Autodesk Inventor part; units mm, degrees
ref_plane "YZ Plane" through (0, 0, 0) normal (1, 0, 0) x (0, 1, 0)
ref_plane "XZ Plane" through (0, 0, 0) normal (0, 1, 0) x (-1, 0, 0)
ref_plane "XY Plane" through (0, 0, 0) normal (0, 0, 1) x (1, 0, 0)
sketch "Skizze2" plane through (0, 0, 0) normal (1, 0, 0) x (0, 1, 0)
  line L0 (0, 0) -> (18.8, 0)
  line L1 (0, 3.1) -> (3, 3.1)
  line L2 (18.8, 31.354) -> (17.3, 31.9)
  line L3 (17.3, 31.9) -> (14.3, 31.9)
  line L4 (14.3, 31.9) -> (14.3, 30.15)
  line L5 (14.3, 30.15) -> (10.8, 30.15)
  line L6 (10.8, 30.15) -> (10.8, 31.9)
  line L7 (10.8, 31.9) -> (7.8, 31.9)
  line L8 (7.8, 31.9) -> (7.8, 35)
  line L9 (7.8, 35) -> (0, 35)
  line L10 (18.8, 31.354) -> (18.8, 27)
  line L11 (18.8, 27) -> (3, 27)
  line L12 (3, 27) -> (3, 3.1)
  line L13 (0, 35) -> (0, 3.1)
  dimension "d5" = 6.2
  dimension "d10" = 20
  dimension "d11" = 60.3
  dimension "d12" = 63.8
  dimension "d26" = 70
  dimension "d34" = 1.5
  dimension "d35" = 4.5
  dimension "d36" = 8
  dimension "d37" = 11
  dimension "d39" = 3
  dimension "d41" = 18.8
  dimension "d50" = 54
revolve "Umdrehung1" add sketch "Skizze2" angle 360 about axis through (0, 0, 0) along (0, 1, 0)
fillet "Rundung1" radius 0.4 2 edges at (0, 10.8, -30.15) (0, 14.3, -30.15)
chamfer "Fase1" distance 0.5 angle 45 1 edges at (0, 0, -3.1)
sketch "Skizze7" plane through (0, 3, 0) normal (0, 1, 0) x (1, 0, 0)
  arc A0 (-7.5, -18.4326) -> (7.5, -18.4326) centre (0, 0) ccw
  circle A1 centre (0, 0) radius 31.9
  line L0 (0, 49) -> (0, -49)
  line L1 (-7.5, -18.4326) -> (-7.5, -25.9374)
  circle A2 centre (0, 0) radius 27
  line L2 (7.5, -18.4326) -> (7.5, -25.9374)
  arc A3 (-7.5, -25.9374) -> (7.5, -25.9374) centre (0, 0) ccw
  line L3 (7.5, 18.4326) -> (7.5, 25.9374)
  arc A4 (7.5, 18.4326) -> (-7.5, 18.4326) centre (0, 0) ccw
  arc A5 (7.5, 25.9374) -> (-7.5, 25.9374) centre (0, 0) ccw
  line L4 (-7.5, 18.4326) -> (-7.5, 25.9374)
  dimension "d70" = 12
  dimension "d73" = 360
  dimension "d75" = 15
extrude "Extrusion2" add sketch "Skizze7" along normal blind 10 contours A0 L0 A2 L1 | A0 L2 A2 L0 | A4 L4 A2 L0 | L0 A2 L3 A4
sketch "Skizze8" plane through (0, 13, 0) normal (0, 1, 0) x (1, 0, 0)
  line L0 (0, 49) -> (0, -49)
  point P0 (0, 0)
  point P1 (0, -23.5)
  dimension "d78" = 23.5
hole "Bohrung3" at (0, 13, 23.5) direction (0, -1, 0) diameter 2.5 depth 8 tip angle 118
thread "Gewinde1"
pattern_circular "Runde Anordnung1" count 2 over 360 about axis through (0, 10.9, 0) along (0, 1, 0) of "Bohrung3"
sketch "Skizze9" plane through (0, 0, 0) normal (0, -1, 0) x (1, 0, 0)
  line L0 (-49, 0) -> (49, 0)
  point P0 (0, 0)
  point P1 (-22, -8)
  point P2 (-22, 8)
  dimension "d91" = 16
  dimension "d92" = 22
hole "Bohrung4" at (-22, 0, -8) at (-22, 0, 8) direction (0, 1, 0) diameter 3.3 end through all
thread "Gewinde2"
thread "Gewinde3"
sketch "Skizze10" plane through (0, 13, 0) normal (0, 1, 0) x (1, 0, 0)
  point P0 (0, 0)
  point P1 (4, -23.5)
  dimension "d104" = 23.5
  dimension "d105" = 4
hole "Bohrung5" at (4, 13, 23.5) direction (0, -1, 0) diameter 0.8 end through all
hole "Bohrung6" at (4, 0, 23.5) direction (0, 1, 0) diameter 1.6 depth 5 tip angle 118
thread "Gewinde4"
sketch "Skizze11" plane through (0, 3, 0) normal (0, 1, 0) x (1, 0, 0)
  line L0 (-49, 0) -> (49, 0)
  point P0 (0, 0)
  point P1 (18.4, 0)
  dimension "d124" = 18.4
hole "Bohrung7" at (18.4, 3, 0) direction (0, -1, 0) diameter 6 end through all
fillet "Rundung2" radius 2 4 edges at (7.5, 8, 25.9374) (-7.5, 8, 25.9374) (7.5, 8, -25.9374) (-7.5, 8, -25.9374)
equation "\"d36\" = d35 + ORing1"
equation "\"ORing1\" = 3.5"
properties part number "Deckel_oben" material "PVC, hart"
Geometry check sheet. Reference: the model listing, model coordinates, mm. A direction names the side the tool comes from. Round coordinates to 2 decimals unless told otherwise and drop trailing zeros. Loops run counter-clockwise (first coordinate to the right, second up) from the corner with the lowest first, then second, coordinate; pieces in that order, holes last. Notation, with made-up numbers: (70.25, 47.25) -> (112.25, 47.25) arc R21 ccw to (112.25, 56.25) -> close; hole circle Ø11 at (45.5, -4.5). An arc over 180 degrees is marked (long way). Use a Markdown table: item, result.
(1) Go/stop test with flat-tipped pins: P1, Ø10, axis at x = 0, z = 0, coming from the +Y side; P2, Ø10, axis at x = -10, y = 2, coming from the +Z side; P3, Ø10, axis at y = 9.5, z = 5.5, coming from the -X side; P4, Ø3.5, axis at x = 18.4, z = 0, coming from the -Y side. Record where each tip stops, or that it passes through.
Calculated:
| item | result |
|---|---|
| P1 | y = 3 |
| P2 | z = 34.64 |
| P3 | x = -34.99 |
| P4 | through |
(2) Mould release check, pull along Z, two halves, no side actions. Record for faces 1 (the flat face through (0, 0, 7)), 2 (the cylindrical face through (21, 4, -28)), 3 (the cylindrical face through (-23.636, 1.521, 8.215)), 4 (the flat face through (7.5, 8, 21)): released by +Z, released by -Z, zero draft, split by the parting line, or undercut.
Calculated:
| item | result |
|---|---|
| face 1 | zero draft |
| face 2 | split by the parting line |
| face 3 | undercut |
| face 4 | undercut |
(3) Sectioned sample at B-B (z = 0). Give the number of separate pieces and of enclosed holes in the cut face, then the cut area to 3 significant figures.
Calculated:
| item | result |
|---|---|
| separate pieces | 3 |
| enclosed holes | 0 |
| area | 345 mm² |
(4) Sectioned sample at A-A (y = 15.5). Enter the section's corners in (x, z).
Calculated:
| item | result |
|---|---|
| outline | circle Ø63.8 at (0, 0); hole circle Ø54 at (0, 0) |
(5) Set-up check for faces 5 (the flat face through (-31, 14.3, 0)), 6 (the cylindrical face through (-8.41, 8.07, 24.8)), 7 (the cylindrical face through (4.306, 2.535, 22.761)): record each of +Z, -Z, +X, -X, +Y, -Y from which the full face is reachable in a straight line by a thin tool's end or side.
Calculated:
| item | result |
|---|---|
| face 5 | none |
| face 6 | +Y |
| face 7 | -Y |
(6) Scan lines: probe 1 along Y at (x, z) = (14.5, 27); probe 2 along Z at (x, y) = (-22, 2); probe 3 along X at (y, z) = (9.5, -23.5). Record each from-to range of solid material in increasing order.
Calculated:
| item | result |
|---|---|
| probe 1 | 0 to 10.8, 14.3 to 18.8 |
| probe 2 | -27.22 to -9.65, -6.35 to 6.35, 9.65 to 27.22 |
| probe 3 | -21.57 to -13.29, -7.54 to -1.25, 1.25 to 7.54, 13.29 to 21.57 |
